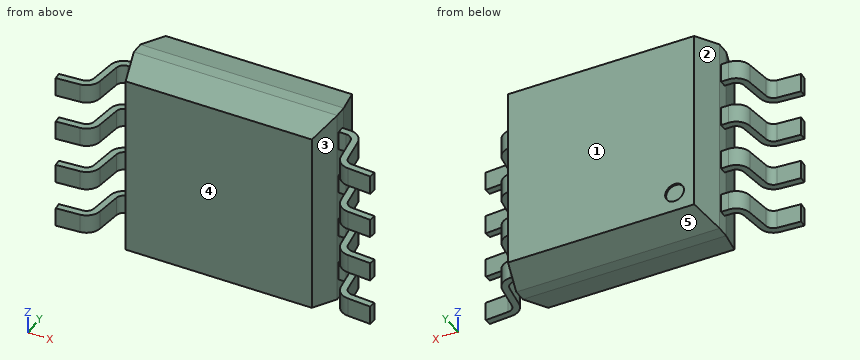
from build123d import *
from OCP.BRepFilletAPI import BRepFilletAPI_MakeChamfer

# Parameters (mm, degrees)
SKETCH1_W              = 5.41
SKETCH1_H              = 5.38
BASE_EXTRUDE_DEPTH     = 2.03
PIN_1_DEPTH            = 0.254
LPATTERN1_COUNT        = 4
LPATTERN1_PITCH        = 1.27
LPATTERN1_COPY_1_DEPTH = 0.254
LPATTERN1_COPY_2_DEPTH = 0.254
LPATTERN1_COPY_3_DEPTH = 0.254
TOP_CHAMFER_SIZE       = 0.85
TOP_CHAMFER_SIZE2      = 0.227756814
BOTTOM_CHAMFER_SIZE    = 0.85
BOTTOM_CHAMFER_SIZE2   = 0.227756814
SKETCH3_R              = 0.25
PIN1_HOL_DEPTH         = 0.05


with BuildPart() as part:
    # Sketch1 → Base-Extrude (new body)
    with BuildSketch(Plane(origin=(0, 0, 0), x_dir=(1, 0, 0), z_dir=(0, 1, 0))):
        Rectangle(SKETCH1_W, SKETCH1_H)
    extrude(amount=-BASE_EXTRUDE_DEPTH)

    # Sketch2 → PIN 1 (add, symmetric)
    with BuildSketch(Plane.XY.offset(-1.905)):
        with BuildLine():
            Line((-2.705, -0.925), (-2.905, -0.925))
            ThreePointArc((-2.905, -0.925), (-3.160863021, -1.020663264), (-3.291204547, -1.260722491))
            Line((-3.291204547, -1.260722491), (-3.38338656, -1.916631596))
            ThreePointArc((-3.38338656, -1.916631596), (-3.448123199, -2.040989522), (-3.576693995, -2.096893695))
            Line((-3.576693995, -2.096893695), (-4.196278083, -2.140219235))
            Line((-4.196278083, -2.140219235), (-4.183721917, -2.319780765))
            Line((-4.183721917, -2.319780765), (-3.56413783, -2.276455225))
            ThreePointArc((-3.56413783, -2.276455225), (-3.325363494, -2.172633189), (-3.205138308, -1.941682754))
            Line((-3.205138308, -1.941682754), (-3.112956294, -1.285773649))
            ThreePointArc((-3.112956294, -1.285773649), (-3.042772396, -1.156510988), (-2.905, -1.105))
            Line((-2.905, -1.105), (-2.705, -1.105))
            Line((-2.705, -1.105), (-2.705, -0.925))
        make_face()
    pin_1 = extrude(amount=PIN_1_DEPTH, both=True)

    # PIN 8: PIN 1 across plane
    add(pin_1.mirror(Plane(origin=(0, 0, 0), x_dir=(0, 0, 1), z_dir=(1, 0, 0))))

    # LPattern1: PIN 1 ×4
    with Locations(*[(0, 0, i * LPATTERN1_PITCH) for i in range(1, LPATTERN1_COUNT)]):
        add(pin_1)

    # LPattern1 copy 1 sketch → LPattern1 copy 1 (add, symmetric)
    with BuildSketch(Plane(origin=(0, 0, -0.635), x_dir=(-1, 0, 0), z_dir=(0, 0, 1))):
        with BuildLine():
            Line((-2.705, 0.925), (-2.905, 0.925))
            ThreePointArc((-2.905, 0.925), (-3.160863021, 1.020663264), (-3.291204547, 1.260722491))
            Line((-3.291204547, 1.260722491), (-3.38338656, 1.916631596))
            ThreePointArc((-3.38338656, 1.916631596), (-3.448123199, 2.040989522), (-3.576693995, 2.096893695))
            Line((-3.576693995, 2.096893695), (-4.196278083, 2.140219235))
            Line((-4.196278083, 2.140219235), (-4.183721917, 2.319780765))
            Line((-4.183721917, 2.319780765), (-3.56413783, 2.276455225))
            ThreePointArc((-3.56413783, 2.276455225), (-3.325363494, 2.172633189), (-3.205138308, 1.941682754))
            Line((-3.205138308, 1.941682754), (-3.112956294, 1.285773649))
            ThreePointArc((-3.112956294, 1.285773649), (-3.042772396, 1.156510988), (-2.905, 1.105))
            Line((-2.905, 1.105), (-2.705, 1.105))
            Line((-2.705, 1.105), (-2.705, 0.925))
        make_face()
    extrude(amount=LPATTERN1_COPY_1_DEPTH, both=True)

    # LPattern1 copy 2 sketch → LPattern1 copy 2 (add, symmetric)
    with BuildSketch(Plane(origin=(0, 0, 0.635), x_dir=(-1, 0, 0), z_dir=(0, 0, 1))):
        with BuildLine():
            Line((-2.705, 0.925), (-2.905, 0.925))
            ThreePointArc((-2.905, 0.925), (-3.160863021, 1.020663264), (-3.291204547, 1.260722491))
            Line((-3.291204547, 1.260722491), (-3.38338656, 1.916631596))
            ThreePointArc((-3.38338656, 1.916631596), (-3.448123199, 2.040989522), (-3.576693995, 2.096893695))
            Line((-3.576693995, 2.096893695), (-4.196278083, 2.140219235))
            Line((-4.196278083, 2.140219235), (-4.183721917, 2.319780765))
            Line((-4.183721917, 2.319780765), (-3.56413783, 2.276455225))
            ThreePointArc((-3.56413783, 2.276455225), (-3.325363494, 2.172633189), (-3.205138308, 1.941682754))
            Line((-3.205138308, 1.941682754), (-3.112956294, 1.285773649))
            ThreePointArc((-3.112956294, 1.285773649), (-3.042772396, 1.156510988), (-2.905, 1.105))
            Line((-2.905, 1.105), (-2.705, 1.105))
            Line((-2.705, 1.105), (-2.705, 0.925))
        make_face()
    extrude(amount=LPATTERN1_COPY_2_DEPTH, both=True)

    # LPattern1 copy 3 sketch → LPattern1 copy 3 (add, symmetric)
    with BuildSketch(Plane(origin=(0, 0, 1.905), x_dir=(-1, 0, 0), z_dir=(0, 0, 1))):
        with BuildLine():
            Line((-2.705, 0.925), (-2.905, 0.925))
            ThreePointArc((-2.905, 0.925), (-3.160863021, 1.020663264), (-3.291204547, 1.260722491))
            Line((-3.291204547, 1.260722491), (-3.38338656, 1.916631596))
            ThreePointArc((-3.38338656, 1.916631596), (-3.448123199, 2.040989522), (-3.576693995, 2.096893695))
            Line((-3.576693995, 2.096893695), (-4.196278083, 2.140219235))
            Line((-4.196278083, 2.140219235), (-4.183721917, 2.319780765))
            Line((-4.183721917, 2.319780765), (-3.56413783, 2.276455225))
            ThreePointArc((-3.56413783, 2.276455225), (-3.325363494, 2.172633189), (-3.205138308, 1.941682754))
            Line((-3.205138308, 1.941682754), (-3.112956294, 1.285773649))
            ThreePointArc((-3.112956294, 1.285773649), (-3.042772396, 1.156510988), (-2.905, 1.105))
            Line((-2.905, 1.105), (-2.705, 1.105))
            Line((-2.705, 1.105), (-2.705, 0.925))
        make_face()
    extrude(amount=LPATTERN1_COPY_3_DEPTH, both=True)

    # TOP CHAMFER: one chamfer whose edges measure the first distance from different faces: ONE call of the kernel's chamfer builder (chamfer() names one face for all edges)
    top_chamfer_edges_1 = [part.edges().sort_by_distance(p)[0] for p in [
        (0, 0, -2.69),
    ]]
    top_chamfer_side_1 = [part.faces().sort_by_distance(p)[0] for p in [
        (0, -1.015, -2.69),
    ]]
    top_chamfer_edges_2 = [part.edges().sort_by_distance(p)[0] for p in [
        (2.705, 0, 0),
    ]]
    top_chamfer_side_2 = [part.faces().sort_by_distance(p)[0] for p in [
        (2.705, -1.015, 0),
    ]]
    top_chamfer_edges_3 = [part.edges().sort_by_distance(p)[0] for p in [
        (0, 0, 2.69),
    ]]
    top_chamfer_side_3 = [part.faces().sort_by_distance(p)[0] for p in [
        (0, -1.015, 2.69),
    ]]
    top_chamfer_edges_4 = [part.edges().sort_by_distance(p)[0] for p in [
        (-2.705, 0, 0),
    ]]
    top_chamfer_side_4 = [part.faces().sort_by_distance(p)[0] for p in [
        (-2.705, -1.015, 0),
    ]]
    top_chamfer = BRepFilletAPI_MakeChamfer(part.part.solid().wrapped)
    for e in top_chamfer_edges_1:
        top_chamfer.Add(TOP_CHAMFER_SIZE, TOP_CHAMFER_SIZE2, e.wrapped, top_chamfer_side_1[0].wrapped)  # the first distance lies on this face
    for e in top_chamfer_edges_2:
        top_chamfer.Add(TOP_CHAMFER_SIZE, TOP_CHAMFER_SIZE2, e.wrapped, top_chamfer_side_2[0].wrapped)  # the first distance lies on this face
    for e in top_chamfer_edges_3:
        top_chamfer.Add(TOP_CHAMFER_SIZE, TOP_CHAMFER_SIZE2, e.wrapped, top_chamfer_side_3[0].wrapped)  # the first distance lies on this face
    for e in top_chamfer_edges_4:
        top_chamfer.Add(TOP_CHAMFER_SIZE, TOP_CHAMFER_SIZE2, e.wrapped, top_chamfer_side_4[0].wrapped)  # the first distance lies on this face
    add(Compound.cast(top_chamfer.Shape()), mode=Mode.REPLACE)

    # BOTTOM CHAMFER: one chamfer whose edges measure the first distance from different faces: ONE call of the kernel's chamfer builder (chamfer() names one face for all edges)
    bottom_chamfer_edges_1 = [part.edges().sort_by_distance(p)[0] for p in [
        (2.705, -2.03, 0),
    ]]
    bottom_chamfer_side_1 = [part.faces().sort_by_distance(p)[0] for p in [
        (2.705, -1.465983178, 0),
    ]]
    bottom_chamfer_edges_2 = [part.edges().sort_by_distance(p)[0] for p in [
        (0, -2.03, -2.69),
    ]]
    bottom_chamfer_side_2 = [part.faces().sort_by_distance(p)[0] for p in [
        (0, -1.44, -2.69),
    ]]
    bottom_chamfer_edges_3 = [part.edges().sort_by_distance(p)[0] for p in [
        (-2.705, -2.03, 0),
    ]]
    bottom_chamfer_side_3 = [part.faces().sort_by_distance(p)[0] for p in [
        (-2.705, -1.465983178, 0),
    ]]
    bottom_chamfer_edges_4 = [part.edges().sort_by_distance(p)[0] for p in [
        (0, -2.03, 2.69),
    ]]
    bottom_chamfer_side_4 = [part.faces().sort_by_distance(p)[0] for p in [
        (0, -1.44, 2.69),
    ]]
    bottom_chamfer = BRepFilletAPI_MakeChamfer(part.part.solid().wrapped)
    for e in bottom_chamfer_edges_1:
        bottom_chamfer.Add(BOTTOM_CHAMFER_SIZE, BOTTOM_CHAMFER_SIZE2, e.wrapped, bottom_chamfer_side_1[0].wrapped)  # the first distance lies on this face
    for e in bottom_chamfer_edges_2:
        bottom_chamfer.Add(BOTTOM_CHAMFER_SIZE, BOTTOM_CHAMFER_SIZE2, e.wrapped, bottom_chamfer_side_2[0].wrapped)  # the first distance lies on this face
    for e in bottom_chamfer_edges_3:
        bottom_chamfer.Add(BOTTOM_CHAMFER_SIZE, BOTTOM_CHAMFER_SIZE2, e.wrapped, bottom_chamfer_side_3[0].wrapped)  # the first distance lies on this face
    for e in bottom_chamfer_edges_4:
        bottom_chamfer.Add(BOTTOM_CHAMFER_SIZE, BOTTOM_CHAMFER_SIZE2, e.wrapped, bottom_chamfer_side_4[0].wrapped)  # the first distance lies on this face
    add(Compound.cast(bottom_chamfer.Shape()), mode=Mode.REPLACE)

    # Sketch3 → PIN1 HOL (cut)
    with BuildSketch(Plane(origin=(0, 0, 0), x_dir=(-1, 0, 0), z_dir=(0, 1, 0))):
        with Locations(Location((1.955, -1.94, 0), (0, 0, 90))):
            Circle(SKETCH3_R)
    extrude(amount=-PIN1_HOL_DEPTH, mode=Mode.SUBTRACT)


solid = part.part
Geometry check sheet. Reference: the model listing, model coordinates, mm. Face numbers are marked on the shaded views. A direction names the side the tool comes from. Round coordinates to 2 decimals unless told otherwise and drop trailing zeros. Loops run counter-clockwise (first coordinate to the right, second up) from the corner with the lowest first, then second, coordinate; pieces in that order, holes last.
Item 1: Access from +Z, -Z, +X, -X, +Y, -Y to the whole of each face (thin tool, end or side, straight path). Record for the marked faces 4 and 5.
Item 2: Thickness scan on line 1 (Z direction, x = 2.75, y = -1.05); line 2 (Y direction, x = 1, z = 1.8); line 3 (Y direction, x = -2.75, z = 1.7) (3 decimals). Record the ranges inside material, lowest first.
Item 3: Cross-section at C-C on y = -0.5. Record the boundary of the cut face in (x, z), then the cut area to 3 significant figures.
Item 4: Mould release check, pull along X, two halves, no side actions. Record for the marked faces 1, 2 and 3: pulls with the +X half, pulls with the -X half, needs draft (parallel to the pull), parting line crosses it, or undercut.
Item 5: Cross-section at A-A on x = 1.75. Record the boundary of the cut face in (y, z).
Item 6: Gauge pin test, flat ends, axial feed: pin 1 (1.1 mm diameter, centred on x = 3.5, y = -1.5, fed in from +Z); pin 2 (1.1 mm diameter, centred on x = -3.5, y = -1.5, fed in from -Z). Record the tip position at first contact, or that the pin passes through.
Answer sheet:
1. face 4: +Z, -Z, -Y
1. face 5: -Z, +X, -X, +Y
2. line 1: z = -2.16 to -1.65, -0.89 to -0.38, 0.38 to 0.89, 1.65 to 2.16
2. line 2: y = -2.03 to 0
2. line 3: y = -1.105 to -0.925
3. outline: (-2.61, -2.6) - (2.61, -2.6) - (2.61, 2.6) - (-2.61, 2.6) - close
3. area: 27.1 mm2
4. face 1: needs draft
4. face 2: pulls with the -X half
4. face 3: undercut
5. outline: (-2.03, -2.46) - (-1.18, -2.69) - (-0.85, -2.69) - (0, -2.46) - (0, 2.46) - (-0.85, 2.69) - (-1.18, 2.69) - (-2.03, 2.46) - close
6. pin 1: stops at z = 2.16
6. pin 2: stops at z = -2.16
